from build123d import *

# Parameters (mm, degrees)
F0_W     = 63.5
F0_H     = 12.7
F0_W_2   = 38.1
F1_DEPTH = 5.08
F2_R     = 14
F3_DEPTH = 2.54
F4_R     = 1.45
F4_R_2   = 2.5
F5_DEPTH = 25.4


with BuildPart() as f1:
    # F0 (on Front) → F1 (new body)
    with BuildSketch(Plane.XZ):
        with Locations((-18.9156212242, -3.6535147662)):
            Rectangle(F0_W, F0_H)
        with Locations((31.8843787758, 9.0464852338)):
            Rectangle(F0_W_2, F0_H)
        with Locations((31.8843787758, -3.6535147662)):
            Rectangle(F0_W_2, F0_H)
        with Locations((82.6843787758, -3.6535147662)):
            Rectangle(F0_W, F0_H)
        with Locations((31.8843787758, -16.3535147662)):
            Rectangle(F0_W_2, F0_H)
    extrude(amount=F1_DEPTH)

    # F2 (on face) → F3 (cut)
    with BuildSketch(Plane.XZ.offset(5.08)):
        with Locations((31.3334800303, -3.4903693013)):
            Circle(F2_R)
    extrude(amount=-F3_DEPTH, mode=Mode.SUBTRACT)

    # F4 (on face) → F5 (cut)
    with BuildSketch(Plane.XZ.offset(2.54)):
        with Locations((39.2787821442, -3.4903693013)):
            Circle(F4_R)
        with Locations((23.2787821442, -3.4903693013)):
            Circle(F4_R)
        with Locations((31.0685478124, -13.1993463289)):
            Circle(F4_R)
        with Locations((31.0685478124, 5.8006536711)):
            Circle(F4_R)
        with Locations((31.3334800303, -3.4903693013)):
            Circle(F4_R_2)
    extrude(amount=-F5_DEPTH, mode=Mode.SUBTRACT)


solid = f1.part
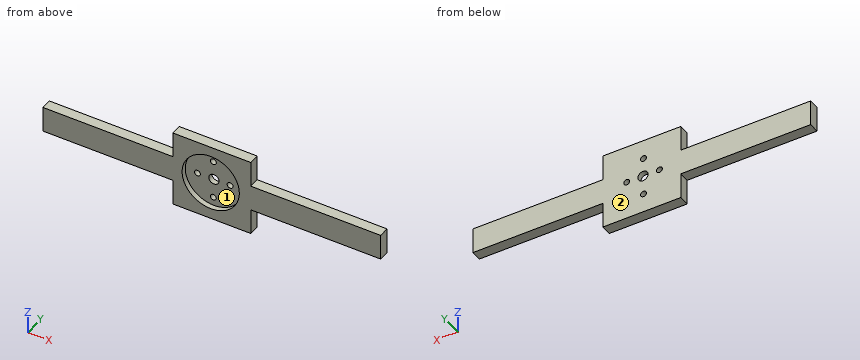
Verification items for the finished model (mm, model axes). Face numbers are marked on the shaded views. Round coordinates to 2 decimals unless told otherwise and drop trailing zeros. Write each loop counter-clockwise with the first axis right and the second up, starting at its lowest first coordinate (ties: lowest second). Pieces come first, ordered by that corner, then holes.
(1) Depth check by flat-ended pin: pin 1 Ø4 at (x, z) = (47.5, -17.5) entering from +Y; pin 2 Ø2.5 at (x, y) = (67.5, -1.5) entering from +Z; pin 3 Ø1.5 at (x, y) = (84, -2) entering from -Z; pin 4 Ø2.5 at (y, z) = (-3, -17) entering from -X. Enter the tip coordinate at first touch or a pass-through.
Returned:
pin 1: stops at y = 0
pin 2: stops at z = 2.7
pin 3: stops at z = -10
pin 4: stops at x = 12.83
(2) Mould release check, pull along X, two halves, no side actions. Record for the marked faces 1 and 2: pulls with the +X half, pulls with the -X half, needs draft (parallel to the pull), parting line crosses it, or undercut.
Returned:
face 1: undercut
face 2: needs draft
(3) Section check A-A (y = -3.5). Enter the section's corners in (x, z), plus the area to 3 significant figures.
Returned:
outline: (-50.67, -10) - (12.83, -10) - (12.83, -22.7) - (50.93, -22.7) - (50.93, -10) - (114.43, -10) - (114.43, 2.7) - (50.93, 2.7) - (50.93, 15.4) - (12.83, 15.4) - (12.83, 2.7) - (-50.67, 2.7) - close; hole circle Ø28 at (31.33, -3.49)
area: 2,450 mm2
(4) Section check B-B (x = 80). Enter the section's corners in (y, z), plus the area to 3 significant figures.
Returned:
outline: (-5.08, -10) - (0, -10) - (0, 2.7) - (-5.08, 2.7) - close
area: 64.5 mm2
(5) Section check C-C (x = 43). Enter the section's corners in (y, z), plus the area to 3 significant figures.
Returned:
outline: (-5.08, -22.7) - (0, -22.7) - (0, 15.4) - (-5.08, 15.4) - (-5.08, 4.25) - (-2.54, 4.25) - (-2.54, -11.23) - (-5.08, -11.23) - close
area: 154 mm2
(6) Material ranges on line 1 (X direction, y = -1.45, z = -4); line 2 (X direction, y = -1.75, z = 9.5); line 3 (Z direction, x = -19, y = -4.05), recorded low to high.
Returned:
line 1: x = -50.67 to 21.92, 24.64 to 28.89, 33.78 to 37.92, 40.64 to 114.43
line 2: x = 12.83 to 50.93
line 3: z = -10 to 2.7
